```python
from build123d import *

# Parameters (mm, degrees)
SKETCH1_R           = 3.5
SKETCH1_R_2         = 2.5
BOSS_EXTRUDE1_DEPTH = 2.8
SKETCH2_R           = 3.5
SKETCH2_R_2         = 1.25
BOSS_EXTRUDE2_DEPTH = 0.2
SKETCH3_R           = 3.5
SKETCH3_R_2         = 2.5
BOSS_EXTRUDE3_DEPTH = 1
BOSS_EXTRUDE4_START = -1.5
BOSS_EXTRUDE4_DEPTH = 1.5


with BuildPart() as part:
    # Sketch1 → Boss-Extrude1 (new body)
    with BuildSketch(Plane.XY):
        Circle(SKETCH1_R)
        Circle(SKETCH1_R_2, mode=Mode.SUBTRACT)
    extrude(amount=BOSS_EXTRUDE1_DEPTH)

    # Sketch2 → Boss-Extrude2 (add)
    with BuildSketch(Plane.XY.offset(2.8)):
        Circle(SKETCH2_R)
        Circle(SKETCH2_R_2, mode=Mode.SUBTRACT)
    extrude(amount=BOSS_EXTRUDE2_DEPTH)

    # Sketch3 → Boss-Extrude3 (add)
    with BuildSketch(Plane.XY.offset(3)):
        Circle(SKETCH3_R)
        Circle(SKETCH3_R_2, mode=Mode.SUBTRACT)
    extrude(amount=BOSS_EXTRUDE3_DEPTH)

    # Sketch4 → Boss-Extrude4 (add)
    with BuildSketch(Plane.XY.offset(4).offset(BOSS_EXTRUDE4_START)):
        with BuildLine():
            Line((-3, -1.802775638), (-1.993465051, -14.223343039))
            ThreePointArc((-1.993465051, -14.223343039), (0, -16.061797098), (1.993465051, -14.223343039))
            Line((1.993465051, -14.223343039), (3, -1.802775638))
            ThreePointArc((3, -1.802775638), (0, -3.5), (-3, -1.802775638))
        make_face()
    boss_extrude4 = extrude(amount=BOSS_EXTRUDE4_DEPTH)

    # Mirror1: Boss-Extrude4 across plane
    add(boss_extrude4.mirror(Plane.ZX))


solid = part.part
```
Here's how the part is built. I have some questions about the finished solid (model axes, mm). A direction names the side the tool comes from. Round coordinates to 2 decimals unless told otherwise and drop trailing zeros. Order: outer loops, then holes, each group sorted by start corner. A loop starts at its lowest first (then second) coordinate and runs counter-clockwise, first axis right, second up. Notation, with made-up numbers: M 79.25,6.5 L 117.25,6.5 A18 cw 117.25,22.5 Z; hole C 37.25,83 d7. An arc over 180 degrees is marked long. Answer in a Markdown table with one row per item.
Item 1: I'm going to push flat-ended pins straight in: pin 1 (1.5 mm diameter, centred on x = 0, y = -1, fed in from +Z); pin 2 (2.5 mm diameter, centred on x = 1, y = 0, fed in from -Z); pin 3 (2 mm diameter, centred on x = 0, y = 0, fed in from -Z). Where does each tip first touch, or does it pass through?
A:
| item | result |
|---|---|
| pin 1 | stops at z = 3 |
| pin 2 | stops at z = 2.8 |
| pin 3 | passes through |
Item 2: Imagine slicing it at C-C, the plane z = 1.9. Write out the boundary of the cut face in (x, y), and give its area (3 significant figures).
A:
| item | result |
|---|---|
| outline | C 0,0 d7; hole C 0,0 d5 |
| area | 18.8 mm2 |
Item 3: Thinking about a two-plate mould opening in Y: for faces 4 (the face through (1, 1, 2.8)), 5 (the face through (3, 0, 4)), 6 (the face through (2.49, -8.1, 3.24)), which applies, +Y half, -Y half, draft (parallel to the pull), parting line (faces both ways), or undercut?
A:
| item | result |
|---|---|
| face 4 | undercut |
| face 5 | draft |
| face 6 | -Y half |
Item 4: If I drill on L1, parallel to Y at x = 0, z = 1.2; L2, parallel to Y at x = 0, z = 2.6; L3, parallel to Z at x = 0.25, y = -6.5, over which ranges is the centre line in solid material (lowest first)? Write a range as from..to.
A:
| item | result |
|---|---|
| L1 | y = -3.5..-2.5, 2.5..3.5 |
| L2 | y = -16.06..-2.5, 2.5..16.06 |
| L3 | z = 2.5..4 |
Item 5: For faces 1 (the face through (-0.54, -2.44, 3.49)), 2 (the face through (3.233, -1.341, 1.528)), 3 (the face through (-0.04, 16.06, 3.24)), which set-ups out of +Z, -Z, +X, -X, +Y, -Y let a thin tool reach every point of the face, with its end or its side?
A:
| item | result |
|---|---|
| face 1 | +Z |
| face 2 | -Z |
| face 3 | +Z, -Z, +Y |
Item 6: Imagine slicing it at D-D, the plane y = 10. Write out the boundary of the cut face in (x, z), and give its area (3 significant figures).
A:
| item | result |
|---|---|
| outline | M -2.34,2.5 L 2.34,2.5 L 2.34,4 L -2.34,4 Z |
| area | 7.01 mm2 |
Item 7: Imagine slicing it at A-A, the plane x = 0. Write out the boundary of the cut face in (y, z), and give its area (3 significant figures).
A:
| item | result |
|---|---|
| outline | M -16.06,2.5 L -3.5,2.5 L -3.5,0 L -2.5,0 L -2.5,2.8 L -1.25,2.8 L -1.25,3 L -2.5,3 L -2.5,4 L -16.06,4 Z; M 1.25,2.8 L 2.5,2.8 L 2.5,0 L 3.5,0 L 3.5,2.5 L 16.06,2.5 L 16.06,4 L 2.5,4 L 2.5,3 L 1.25,3 Z |
| area | 46.2 mm2 |
Item 8: Imagine slicing it at B-B, the plane y = 0. Write out the boundary of the cut face in (x, z).
A:
| item | result |
|---|---|
| outline | M -3.5,0 L -2.5,0 L -2.5,2.8 L -1.25,2.8 L -1.25,3 L -2.5,3 L -2.5,4 L -3.5,4 Z; M 1.25,2.8 L 2.5,2.8 L 2.5,0 L 3.5,0 L 3.5,4 L 2.5,4 L 2.5,3 L 1.25,3 Z |
